Check sheet for the modelled part. Datum: model origin and axes. Units: mm. Face numbers are marked on the shaded views. A direction names the side the tool comes from. Give positions to 0.01 mm unless a question says otherwise; leave off trailing zeros. Loops run counter-clockwise (first coordinate to the right, second up) from the corner with the lowest first, then second, coordinate; pieces in that order, holes last. Notation, with made-up numbers: M 62.25,83.5 L 95.25,83.5 A24 cw 95.25,116.5 Z; hole C 42.25,16 d3. An arc over 180 degrees is marked long. Write each question's results on one line, items separated by ' | '. Start each with the question number.
1. Sectioned sample at D-D on z = 7. Record the cut outline in (x, y).
2. Go/stop test with flat-tipped pins: pin 1 (2.5 mm diameter, centred on x = 1, y = -1.5, fed in from -Z); pin 2 (5 mm diameter, centred on x = 6.5, z = 7, fed in from -Y); pin 3 (3 mm diameter, centred on y = -2, z = 7, fed in from -X); pin 4 (3 mm diameter, centred on x = 0, y = -1.5, fed in from +Z). Record where each tip stops, or that it passes through.
3. Draft check along X on the marked faces 1, 2, 3 and 4. Enter one of: pulls with the +X half, pulls with the -X half, needs draft (parallel to the pull), parting line crosses it, or undercut.
4. Sectioned sample at A-A on z = 23. Record the cut outline in (x, y), and give its area (3 significant figures).
5. Sectioned sample at C-C on x = 0. Record the cut outline in (y, z).
6. Material ranges on line 1 along Z through (x, y) = (6.5, -3.05); line 2 along X through (y, z) = (-1.8, 7); line 3 along X through (y, z) = (2.3, 23), recorded low to high.
7. Tool access check on the marked faces 5, 6, 7, 8 and 9. Record the directions out of +Z, -Z, +X, -X, +Y, -Y that give a thin tool (end or side, any length) a straight path to the whole face; none if there is none.
8. Sectioned sample at B-B on y = 0. Record the cut outline in (x, z).
```python
from build123d import *

# Parameters (mm, degrees)
CYLINDER010_R            = 2.75
CYLINDER010_DEPTH        = 20
PRISM002_DEPTH           = 20
PRISM002_PLACEMENT_ANGLE = 30
CYLINDER009_R            = 1.5
CYLINDER009_DEPTH        = 20
FUSION009_ROLL_ANGLE     = 90
FUSION008_ROLL_ANGLE     = 90
BOX001_W                 = 13
BOX001_H                 = 2
BOX001_DEPTH             = 32
CYLINDER008_R            = 2.5
CYLINDER008_DEPTH        = 32
CYLINDER007_R            = 4
CYLINDER007_DEPTH        = 16
CYLINDER006_R            = 10
CYLINDER006_DEPTH        = 30
CHAMFER003_SIZE          = 0.4


with BuildPart() as cylinder010:
    # Cylinder010 → Cylinder010 (new body)
    with BuildSketch(Plane.XY.offset(4)):
        Circle(CYLINDER010_R)
    extrude(amount=CYLINDER010_DEPTH)


with BuildPart() as prism002:
    # Prism002 → Prism002 (new body)
    with BuildSketch(Plane.XY):
        Polygon((3.2, 0), (1.6, 2.771281), (-1.6, 2.771281), (-3.2, 0), (-1.6, -2.771281), (1.6, -2.771281), align=None)
    extrude(amount=PRISM002_DEPTH)


with BuildPart() as prism002_1:
    # Prism002 placement: moved
    add(prism002.part.moved(Location((0, 0, -24))).rotate(Axis((0, 0, -24), (0, 0, 1)), PRISM002_PLACEMENT_ANGLE))


with BuildPart() as cylinder009:
    # Cylinder009 → Cylinder009 (new body)
    with BuildSketch(Plane.XY.offset(-7)):
        Circle(CYLINDER009_R)
    extrude(amount=CYLINDER009_DEPTH)


with BuildPart() as fusion009:
    # Fusion009 base: copy of Cylinder009
    add(cylinder009.part)

    # Fusion009: union Cylinder010, Prism002
    add(cylinder010.part)
    add(prism002_1.part)


with BuildPart() as fusion009_1:
    # Fusion009 roll: moved
    add(fusion009.part.rotate(Axis((0, 0, 0), (1, 0, 0)), FUSION009_ROLL_ANGLE))


with BuildPart() as fusion009_2:
    # Fusion009 placement: moved
    add(fusion009_1.part.moved(Location((6.5, 0, 23))))


with BuildPart() as fusion010:
    # Fusion008 base: copy of Cylinder009
    add(cylinder009.part)

    # Fusion008: union Cylinder010, Prism002
    add(cylinder010.part)
    add(prism002_1.part)


with BuildPart() as fusion010_1:
    # Fusion008 roll: moved
    add(fusion010.part.rotate(Axis((0, 0, 0), (1, 0, 0)), FUSION008_ROLL_ANGLE))


with BuildPart() as fusion010_2:
    # Fusion008 placement: moved
    add(fusion010_1.part.moved(Location((6.5, 0, 7))))

    # Fusion010: union Fusion009
    add(fusion009_2.part)


with BuildPart() as cube001:
    # Box001 → Box001 (new body)
    with BuildSketch(Plane(origin=(0, -1, -1), x_dir=(1, 0, 0), z_dir=(0, 0, 1))):
        with Locations((6.5, 1)):
            Rectangle(BOX001_W, BOX001_H)
    extrude(amount=BOX001_DEPTH)


with BuildPart() as cylinder008:
    # Cylinder008 → Cylinder008 (new body)
    with BuildSketch(Plane.XY.offset(-1)):
        Circle(CYLINDER008_R)
    extrude(amount=CYLINDER008_DEPTH)


with BuildPart() as fusion007:
    # Cylinder007 → Cylinder007 (new body)
    with BuildSketch(Plane.XY.offset(-1)):
        Circle(CYLINDER007_R)
    extrude(amount=CYLINDER007_DEPTH)

    # Fusion007: union Cube001, Cylinder008
    add(cube001.part)
    add(cylinder008.part)


with BuildPart() as chamfer003:
    # Cylinder006 → Cylinder006 (new body)
    with BuildSketch(Plane.XY):
        Circle(CYLINDER006_R)
    extrude(amount=CYLINDER006_DEPTH)

    # Cut005: cut Fusion007
    add(fusion007.part, mode=Mode.SUBTRACT)

    # Cut006: cut Fusion010
    add(fusion010_2.part, mode=Mode.SUBTRACT)

    # Chamfer003
    chamfer003_edges = [chamfer003.edges().sort_by_distance(p)[0] for p in [
        (-2.5, 0, 30),
        (3.872983, 1, 7.5),
        (2.291288, 1, 22.5),
        (3.872983, -1, 7.5),
        (2.291288, -1, 22.5),
        (-4, 0, 0),
    ]]
    chamfer(chamfer003_edges, length=CHAMFER003_SIZE)


solid = chamfer003.part
```
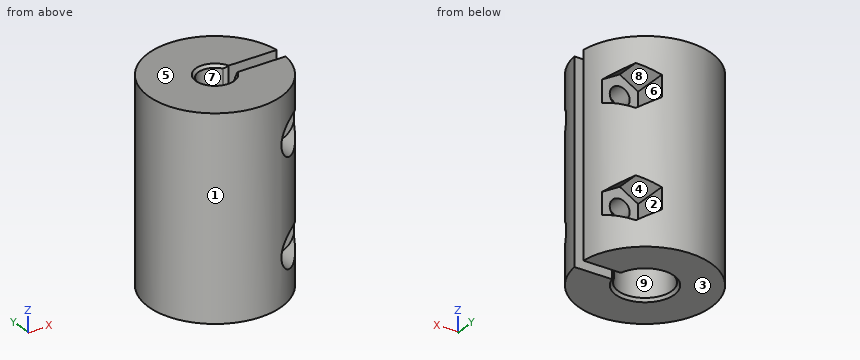
Output values:
1) outline: M 3.73,4 L 3.73,9.28 A10 ccw long 3.75,-9.27 L 3.75,-4 L 5,-4 L 5,-1 L 4.27,-1 L 3.75,-1.38 A4 cw long 3.75,1.38 L 4.27,1 L 5,1 L 5,4 Z; M 8,-4 L 9.17,-4 A10 ccw 9.95,-1 L 8,-1 Z; M 8,1 L 9.95,1 A10 ccw 9.17,4 L 8,4 Z
2) pin 1: z = 15 | pin 2: y = -4 | pin 3: x = -9.99 | pin 4: z = 30
3) face 1: parting line crosses it | face 2: pulls with the +X half | face 3: needs draft | face 4: undercut
4) outline: M 2.1,-1.35 A2.5 cw long 2.1,1.35 L 2.69,1 L 5,1 L 5,4 L 3.73,4 L 3.73,9.28 A10 ccw long 3.75,-9.27 L 3.75,-4 L 5,-4 L 5,-1 L 2.69,-1 Z; M 8,-4 L 9.17,-4 A10 ccw 9.95,-1 L 8,-1 Z; M 8,1 L 9.95,1 A10 ccw 9.17,4 L 8,4 Z | area: 225 mm2
5) outline: M -10,0 L -4.4,0 L -4,0.4 L -4,15 L -2.5,15 L -2.5,29.6 L -2.9,30 L -10,30 Z; M 2.5,15 L 4,15 L 4,0.4 L 4.4,0 L 10,0 L 10,30 L 2.9,30 L 2.5,29.6 Z
6) line 1: 0 to 5.5, 8.5 to 21.5, 24.5 to 30 | line 2: -9.84 to -3.57, 3.57 to 5, 8 to 9.84 | line 3: -9.73 to -0.98, 0.98 to 5, 8 to 9.73
7) face 5: +Z, +X, -X, +Y, -Y | face 6: +X, +Y | face 7: +Z, -Z | face 8: +Y | face 9: -Z
8) outline: M -10,0 L -4.4,0 L -4,0.4 L -4,15 L -2.5,15 L -2.5,29.6 L -2.9,30 L -10,30 Z
